Geometry: see drawing. Coordinates: mm, zero at the bounding-box minimum. A direction names the side the tool comes from. Give positions to 0.01 mm unless a question says otherwise; leave off trailing zeros. Write each loop counter-clockwise with the first axis right and the second up, starting at its lowest first coordinate (ties: lowest second). Pieces come first, ordered by that corner, then holes. Notation, with made-up numbers: M -35.75,51.25 L 13.25,51.25 A13 cw 13.25,66.25 Z; hole C 58,6.5 d5. An arc over 180 degrees is marked long. Use CSV: the item, a comma, the result in double quotes. Start each with the question number.
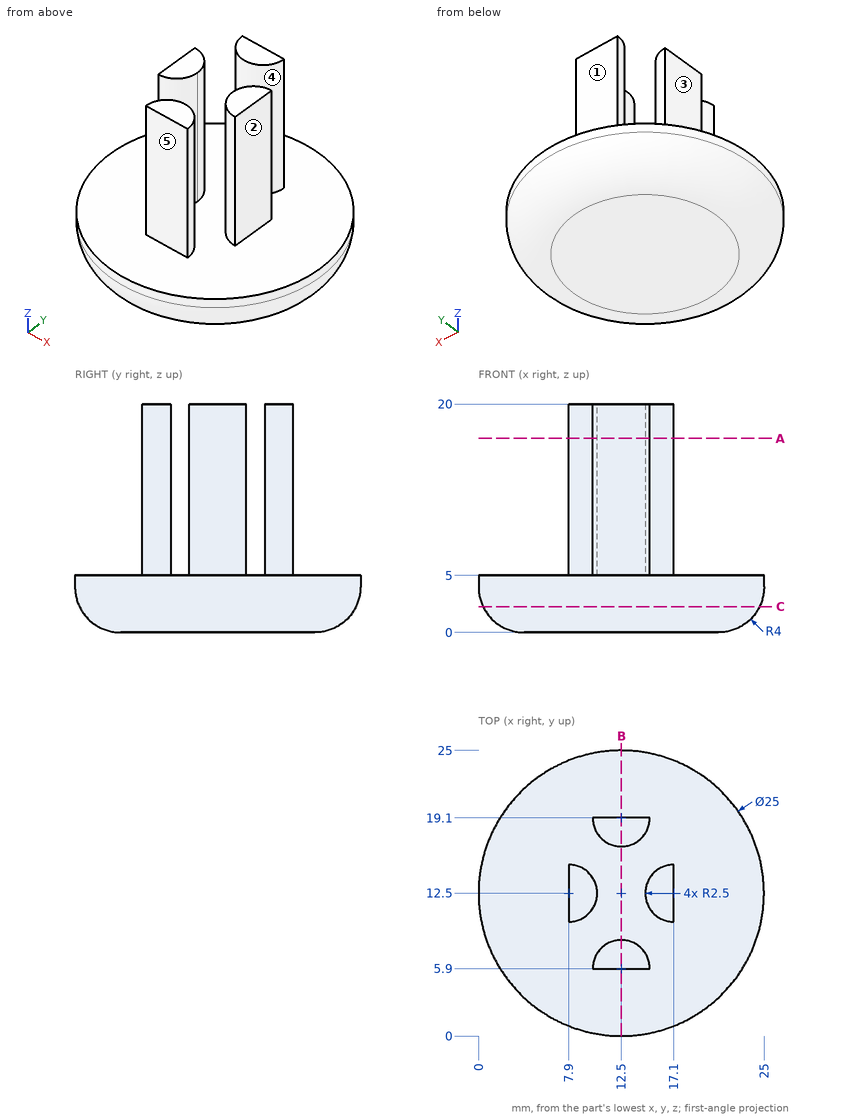
1. Section C-C on z = 2.25. Return loops of the section in (x, y), then the cut area to 3 significant figures.
2. First-contact query: pin 1 (1.5 mm diameter, centred on y = 12.5, z = 13, fed in from -X); pin 2 (5 mm diameter, centred on x = 17, z = 4, fed in from -Y); pin 3 (5.5 mm diameter, centred on y = 12.5, z = 14.5, fed in from +X). Flat tips, straight axial feed; report the tip coordinate or a pass-through.
3. Line query: probe 1 along Y at (x, z) = (14.5, 15); probe 2 along X at (y, z) = (12.5, 14.75); probe 3 along Z at (x, y) = (11.5, 11.25). Output: solid intervals per line, ascending.
4. Access query for the marked faces 1, 2, 3, 4 and 5. Directions: +Z, -Z, +X, -X, +Y, -Y. A direction counts if a zero-diameter tool reaches every point of the face in a straight line with its end or side. Return the directions, or none.
5. Section A-A on z = 17. Return loops of the section in (x, y), then the cut area to 3 significant figures.
6. Section B-B on x = 12.5. Return loops of the section in (y, z).
Resolved:
1,outline,"C 12.5,12.5 d24.19"
1,area,"460 mm2"
2,pin 1,"stops at x = 7.9"
2,pin 2,"stops at y = 0.16"
2,pin 3,"stops at x = 17.1"
3,probe 1,"y = 5.9 to 7.4, 17.6 to 19.1"
3,probe 2,"x = 7.9 to 10.4, 14.6 to 17.1"
3,probe 3,"z = 0 to 5"
4,face 1,"+Z, +X, -X, +Y"
4,face 2,"+Z, +X, +Y, -Y"
4,face 3,"+Z, -X, +Y, -Y"
4,face 4,"+Z"
4,face 5,"+Z, +X, -X, -Y"
5,outline,"M 7.9,10 A2.5 ccw 7.9,15 Z; M 10,5.9 L 15,5.9 A2.5 ccw Z; M 10,19.1 A2.5 ccw 15,19.1 Z; M 17.1,10 L 17.1,15 A2.5 ccw Z"
5,area,"39.3 mm2"
6,outline,"M 0,4 A4 ccw 4,0 L 21,0 A4 ccw 25,4 L 25,5 L 19.1,5 L 19.1,20 L 16.6,20 L 16.6,5 L 8.4,5 L 8.4,20 L 5.9,20 L 5.9,5 L 0,5 Z"
